Can you work these out from the model? Positions are in its coordinate system, mm. A direction names the side the tool comes from. Round coordinates to 2 decimals unless told otherwise and drop trailing zeros. Order: outer loops, then holes, each group sorted by start corner. A loop starts at its lowest first (then second) coordinate and runs counter-clockwise, first axis right, second up.
Q1. If we section it at C-C (x = 63): Please give me the cut outline in (y, z).
Q2. Will these pins go through, and if not, where does the flat tip stop? P1, Ø1.5, axis at x = -40.5, z = 4.5, coming from the -Y side; P2, Ø2, axis at x = -49, z = 1, coming from the -Y side; P3, Ø7.5, axis at x = -84.5, y = 18.5, coming from the +Z side.
Q3. If I drill on line 1 (Y direction, x = -82.4, z = 0.15); line 2 (Y direction, x = -55, z = 0.25); line 3 (Y direction, x = 62.5, z = 3.25), over which ranges is the centre line in solid material (lowest first)?
Q4. We'd pull the mould along X, two halves only. Please class faces 1 (the face through (53, -27, 1)), 2 (the face through (92.4, -18, 1)), 3 (the face through (83.974, -17.004, 0.921)), 4 (the face through (-80.826, 17.996, 0.379)): pulls with the +X half, pulls with the -X half, needs draft (parallel to the pull), parting line crosses it, or undercut.
Q5. If we section it at A-A (x = 82.4): Please give me the cut outline in (y, z), plus the area to 3 significant figures.
Q6. For faces 5 (the face through (48, -11.1, 4)), 6 (the face through (-46, 11.1, 4)), 7 (the face through (-57, 6.9, 1)), 8 (the face through (44, -23.9, 4)), which set-ups out of +Z, -Z, +X, -X, +Y, -Y let a thin tool reach every point of the face, with its end or its side?
Q7. If we section it at D-D (z = 4.75): Please give me the cut outline in (x, y).
Q8. If we section it at B-B (y = 17.5): Please give me the cut outline in (x, z), plus the area to 3 significant figures.
from build123d import *

# Parameters (mm, degrees)
SKETCH_1_R          = 1.65
EXTRUDE_1_DEPTH     = 3
EXTRUDE_2_DEPTH     = 2.9
CHAMFER_1_SIZE      = 2.9
EXTRUDE_START       = -1.1
SKETCH_6_R          = 1.65
EXTRUDE_3_DEPTH     = 4.1
CUT_EXTRUDE_START   = 3
SKETCH_7_W          = 21
SKETCH_7_H          = 15.2
CUT_EXTRUDE_1_DEPTH = 1.1
FILLET_1_R          = 1


with BuildPart() as part:
    # 草图1 → 凸台-拉伸1 (new body)
    with BuildSketch(Plane.XY):
        Polygon((-92.4, 27), (-13.564971157, 27), (21.435028843, -8), (92.4, -8), (92.4, -27), (13.564971157, -27), (-21.435028843, 8), (-92.4, 8), align=None)
        with Locations((-82.4, 17.5)):
            Circle(SKETCH_1_R, mode=Mode.SUBTRACT)
        with Locations((82.4, -17.5)):
            Circle(SKETCH_1_R, mode=Mode.SUBTRACT)
    extrude(amount=EXTRUDE_1_DEPTH)

    # 草图2 → 凸台-拉伸2 (add)
    with BuildSketch(Plane.XY.offset(3)):
        Polygon((-71.4, 23.9), (-71.4, 11.1), (-19.150966799, 11.1), (15.849033201, -23.9), (73.4, -23.9), (73.4, -11.1), (21.150966799, -11.1), (-13.849033201, 23.9), align=None)
    extrude(amount=EXTRUDE_2_DEPTH)

    # 倒角1
    chamfer_1_edges = [part.edges().sort_by_distance(p)[0] for p in [
        (73.4, -17.5, 5.9),
        (-71.4, 17.5, 5.9),
    ]]
    chamfer(chamfer_1_edges, length=CHAMFER_1_SIZE - 0.0001)  # a hair under: the kernel refuses the full size

    # 草图6 → 凸台-拉伸3 (add)
    with BuildSketch(Plane.XY.offset(EXTRUDE_START)):
        Polygon((-92.4, 28.1), (-92.4, 6.9), (-20.335028843, 6.9), (13.564971157, -27), (92.4, -27), (92.4, -8), (21.435028843, -8), (-14.664971157, 28.1), align=None)
        with Locations((-82.4, 17.5)):
            Circle(SKETCH_6_R, mode=Mode.SUBTRACT)
        with Locations((82.4, -17.5)):
            Circle(SKETCH_6_R, mode=Mode.SUBTRACT)
    extrude(amount=EXTRUDE_3_DEPTH)

    # 草图7 → 切除-拉伸1 (cut)
    with BuildSketch(Plane.XY.offset(CUT_EXTRUDE_START)):
        with Locations((-81.9, 17.5)):
            Rectangle(SKETCH_7_W, SKETCH_7_H)
    extrude(amount=-CUT_EXTRUDE_1_DEPTH, mode=Mode.SUBTRACT)

    # 圆角1
    fillet_1_edges = [part.edges().sort_by_distance(p)[0] for p in [
        (21.435028843, -8, 0.95),
        (13.564971157, -27, 0.95),
        (-13.849033201, 23.9, 4.45),
        (-19.150966799, 11.1, 4.45),
        (15.849033201, -23.9, 4.45),
        (21.150966799, -11.1, 4.45),
        (-14.664971157, 28.1, 0.95),
        (-20.335028843, 6.9, 0.95),
    ]]
    fillet(fillet_1_edges, radius=FILLET_1_R)


solid = part.part
Solution:
1. outline: (-27, -1.1) - (-8, -1.1) - (-8, 3) - (-11.1, 3) - (-11.1, 5.9) - (-23.9, 5.9) - (-23.9, 3) - (-27, 3) - close
2. P1: stops at y = 11.1
2. P2: stops at y = 6.9
2. P3: stops at z = 1.9
3. line 1: y = 6.9 to 15.85, 19.15 to 28.1
3. line 2: y = 6.9 to 28.1
3. line 3: y = -23.9 to -11.1
4. face 1: needs draft
4. face 2: pulls with the +X half
4. face 3: undercut
4. face 4: undercut
5. outline: (-27, -1.1) - (-19.15, -1.1) - (-19.15, 3) - (-27, 3) - close; (-15.85, -1.1) - (-8, -1.1) - (-8, 3) - (-15.85, 3) - close
5. area: 64.4 mm2
6. face 5: +Z, +X, +Y
6. face 6: +Z, -X, -Y
6. face 7: +Z, -Z, -X, -Y
6. face 8: +Z, +X, -X, -Y
7. outline: (-69.65, 11.1) - (-19.57, 11.1) arc R1 cw to (-18.86, 10.81) - (15.56, -23.61) arc R1 ccw to (16.26, -23.9) - (71.65, -23.9) - (71.65, -11.1) - (21.57, -11.1) arc R1 cw to (20.86, -10.81) - (-13.56, 23.61) arc R1 ccw to (-14.26, 23.9) - (-69.65, 23.9) - close
8. outline: (-92.4, -1.1) - (-84.05, -1.1) - (-84.05, 1.9) - (-92.4, 1.9) - close; (-80.75, -1.1) - (-4.06, -1.1) - (-4.06, 3) - (-7.45, 3) - (-7.45, 5.9) - (-68.5, 5.9) - (-71.4, 3) - (-71.4, 1.9) - (-80.75, 1.9) - close
8. area: 510 mm2
